Check sheet for the drawn part. Datum: minimum x, y, z corner. Units: mm. Coordinates: 2 decimals unless noted, no trailing zeros. Loops run counter-clockwise (first coordinate to the right, second up) from the corner with the lowest first, then second, coordinate; pieces in that order, holes last.
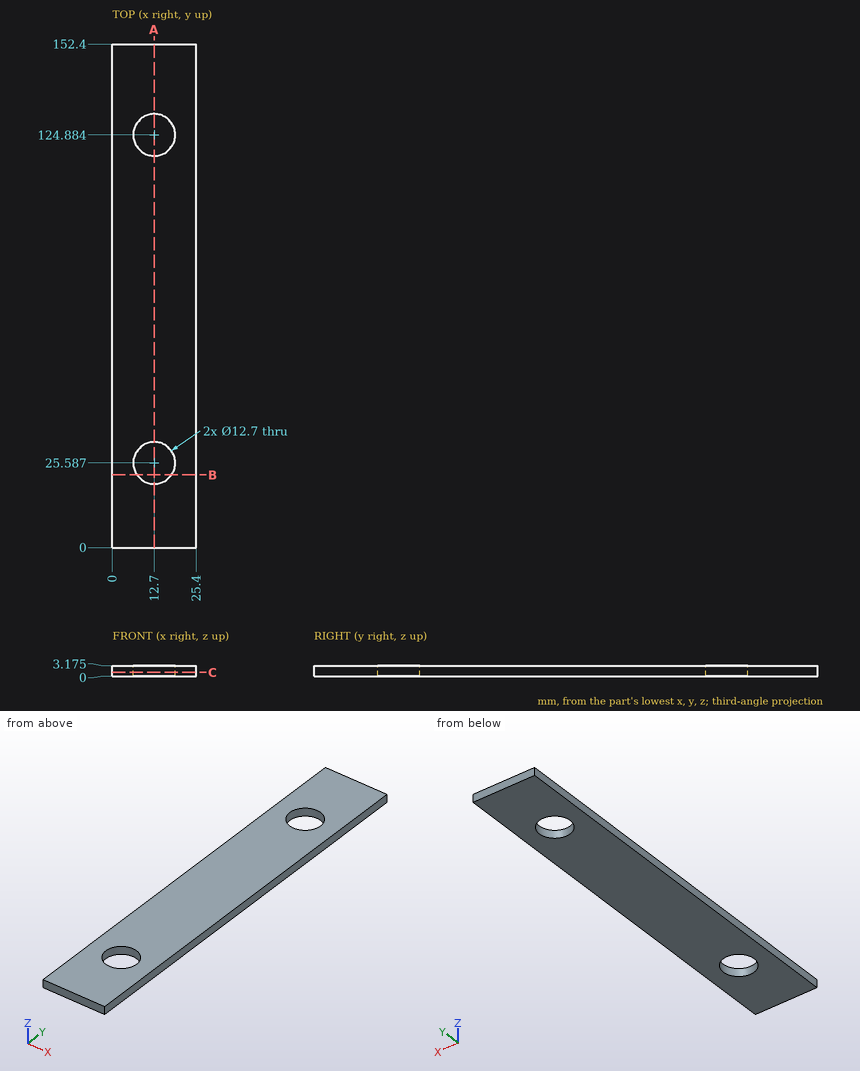
(1) Scan lines: L1, parallel to Y at x = 12.7, z = 1.8 (1 decimal); L2, parallel to X at y = 25, z = 0.9; L3, parallel to X at y = 31, z = 1.85. Record each from-to range of solid material in increasing order.
Findings:
L1: y = 0 to 19.2, 31.9 to 118.5, 131.2 to 152.4
L2: x = 0 to 6.38, 19.02 to 25.4
L3: x = 0 to 9.38, 16.02 to 25.4
(2) Sectioned sample at A-A on x = 12.7. Record the cut outline in (y, z) (1 decimal), and give its area (3 significant figures).
Findings:
outline: (0, 0) - (19.2, 0) - (19.2, 3.2) - (0, 3.2) - close; (31.9, 0) - (118.5, 0) - (118.5, 3.2) - (31.9, 3.2) - close; (131.2, 0) - (152.4, 0) - (152.4, 3.2) - (131.2, 3.2) - close
area: 403 mm2
(3) Sectioned sample at C-C on z = 1.1. State how many separate pieces and enclosed holes the cut face has, and give its area (3 significant figures).
Findings:
separate pieces: 1
enclosed holes: 2
area: 3,620 mm2
(4) Sectioned sample at B-B on y = 22. Record the cut outline in (x, z) (1 decimal).
Findings:
outline: (0, 0) - (7.5, 0) - (7.5, 3.2) - (0, 3.2) - close; (17.9, 0) - (25.4, 0) - (25.4, 3.2) - (17.9, 3.2) - close
